```python
from build123d import *

# Parameters (mm, degrees)
F1_DEPTH = 203.2
F2_R     = 5.08
F4_DEPTH = 508
F5_R     = 17.4625
F6_DEPTH = 152.4
F8_DEPTH = 508


with BuildPart() as f1:
    # F0 (on Front) → F1 (new body)
    with BuildSketch(Plane.XZ):
        Polygon((-76.2, -46.21704), (-76.2, -57.094753), (76.2, -57.094753), (76.2, -46.21704), (26.83735, -33.72637), (21.163462, -31.835258), (18.708812, -29.612178), (16.218112, -26.55388), (14.689744, -22.895062), (13.485576, -19.143616), (13.305501, -16.85449), (10.935693, -2.660843), (9.173225, 23.941404), (9.095304, 51.274587), (9.465817, 61.371074), (10.203332, 68.52603), (11.415046, 73.405639), (12.987001, 77.66302), (14.984693, 80.446691), (18.095852, 83.001115), (20.683027, 84.147327), (25.922873, 85.98128), (30.180251, 87.1275), (33.094916, 87.749728), (34.175634, 88.306465), (35.387348, 89.616426), (36.173157, 90.991981), (36.40228, 91.97448), (36.598587, 93.513711), (36.598872, 93.52041), (36.827176, 98.88458), (36.669851, 103.667696), (36.407496, 106.64783), (36.177806, 110.315693), (35.555092, 114.278253), (34.24468, 117.978737), (33.327476, 119.878062), (31.132972, 122.464971), (28.218115, 124.036569), (24.026078, 125.34602), (19.539378, 126.000454), (15.433662, 126.392808), (7.999516, 126.762047), (0, 126.762047), (-7.999516, 126.762047), (-15.433662, 126.392808), (-19.539378, 126.000454), (-24.026078, 125.34602), (-28.218115, 124.036569), (-31.132972, 122.464971), (-33.327476, 119.878062), (-34.24468, 117.978737), (-35.555092, 114.278253), (-36.177806, 110.315693), (-36.407496, 106.64783), (-36.669851, 103.667696), (-36.827176, 98.88458), (-36.598872, 93.52041), (-36.598587, 93.513711), (-36.40228, 91.97448), (-36.173157, 90.991981), (-35.387348, 89.616426), (-34.175634, 88.306465), (-33.094916, 87.749728), (-30.180251, 87.1275), (-25.922873, 85.98128), (-20.683027, 84.147327), (-18.095852, 83.001115), (-14.984693, 80.446691), (-12.987001, 77.66302), (-11.415046, 73.405639), (-10.203332, 68.52603), (-9.465817, 61.371074), (-9.095304, 51.274587), (-9.173225, 23.941404), (-10.935693, -2.660843), (-13.305501, -16.85449), (-13.485576, -19.143616), (-14.689744, -22.895062), (-16.218112, -26.55388), (-18.708812, -29.612178), (-21.163462, -31.835258), (-26.83735, -33.72637), align=None)
    extrude(amount=F1_DEPTH)

    # F2
    f2_edges = [f1.edges().sort_by_distance(p)[0] for p in [
        (76.2, -101.6, -46.21704),
        (-76.2, -101.6, -46.21704),
    ]]
    fillet(f2_edges, radius=F2_R)

    # F3 (on face) → F4 (cut)
    with BuildSketch(Plane.XZ.offset(203.2)):
        with BuildLine():
            Line((26.83735, -33.72637), (21.163462, -31.835258))
            Line((21.163462, -31.835258), (21.163462, -57.094753))
            Line((21.163462, -57.094753), (76.2, -57.094753))
            Line((76.2, -57.094753), (76.2, -50.171713))
            ThreePointArc((76.2, -50.171713), (75.128547, -47.051144), (72.366162, -45.24693))
            Line((72.366162, -45.24693), (26.83735, -33.72637))
        make_face()
    extrude(amount=-F4_DEPTH, mode=Mode.SUBTRACT)

    # F5 (on Right) → F6 (cut, symmetric)
    with BuildSketch(Plane.YZ):
        with Locations((-101.6, 37.607995)):
            Circle(F5_R)
    extrude(amount=F6_DEPTH, both=True, mode=Mode.SUBTRACT)

    # F7 (on face) → F8 (cut)
    with BuildSketch(Plane.XZ.offset(203.2)):
        Polygon((15.433662, 126.392808), (7.999516, 126.762047), (36.669851, 103.667696), (36.407496, 106.64783), (36.177806, 110.315693), (35.555092, 114.278253), (34.24468, 117.978737), (33.327476, 119.878062), (31.132972, 122.464971), (28.218115, 124.036569), (24.026078, 125.34602), (19.539378, 126.000454), align=None)
    extrude(amount=-F8_DEPTH, mode=Mode.SUBTRACT)


solid = f1.part
```
The listing builds one solid part. Answer for the finished solid, in the listing's coordinates (mm). A direction names the side the tool comes from. Coordinates: 2 decimals unless noted, no trailing zeros. Write each loop counter-clockwise with the first axis right and the second up, starting at its lowest first coordinate (ties: lowest second). Pieces come first, ordered by that corner, then holes. Notation, with made-up numbers: M -16.75,3 L 2.25,3 A14 cw 2.25,17 Z; hole C -24,26 d6. An arc over 180 degrees is marked long. Use a Markdown table: item, result. Add a question column.
1. For a pull along Z with two mould halves and no side action, classify faces 5 (the flat face through (-8, -203.2, 36)), 6 (the flat face through (10.8, -100.18, 70.93)), 7 (the cylindrical face through (-75.16, -103.02, -47.09)) as +Z half, -Z half, draft (parallel to the pull), parting line (faces both ways), or undercut.
2. Straight lines are drawn through the part: line 1 along Z through (x, y) = (1.5, -101.6); line 2 along X through (y, z) = (-55.5, 41); line 3 along Z through (x, y) = (2, -101). For each, find the intervals that lie inside material, in ascending order. Write a range as [from, to].
3. Section A-A (x = -47.5) is taken. Give the vertices of the cut face in (y, z).
4. Section B-B (z = 1.5) is taken. Give the vertices of the cut face in (x, y), plus the area to 3 significant figures.
5. Which of the six approach directions +Z, -Z, +X, -X, +Y, -Y give full straight-line access (tool end or side, diameter ignored) to faces 1 (the flat face through (-21.75, -100.18, 125.68)), 2 (the flat face through (-49.283, -100.178, -39.406)), 3 (the flat face through (10.067, -100.178, 10.454)), 4 (the flat face through (21.163, -103, -44))?
6. Given P1, Ø2, axis at x = -24.5, y = -35, coming from the +Z side; P2, Ø2, axis at x = 17, z = -24, coming from the +Y side; P3, Ø5, axis at y = -55.5, z = 45.5, coming from the +X side; P4, Ø1, axis at y = -76.5, z = 105.5, coming from the -X side, each flat-ended and moving along its own axis, determine where each tip first touches the part or whether it passes through.
Data:
| question | item | result |
|---|---|---|
| 1 | face 5 | draft |
| 1 | face 6 | undercut |
| 1 | face 7 | +Z half |
| 2 | line 1 | z = [-57.09, 20.15], [55.07, 126.76] |
| 2 | line 2 | x = [-9.12, 9.12] |
| 2 | line 3 | z = [-57.09, 20.16], [55.06, 126.76] |
| 3 | outline | M -203.2,-57.09 L 0,-57.09 L 0,-38.95 L -203.2,-38.95 Z |
| 4 | outline | M -10.66,-203.2 L 10.66,-203.2 L 10.66,0 L -10.66,0 Z |
| 4 | area | 4,330 mm2 |
| 5 | face 1 | +Z, -X, +Y, -Y |
| 5 | face 2 | -X, +Y, -Y |
| 5 | face 3 | +X, +Y, -Y |
| 5 | face 4 | -Z, +X, +Y, -Y |
| 6 | P1 | stops at z = 125.42 |
| 6 | P2 | passes through |
| 6 | P3 | stops at x = 9.12 |
| 6 | P4 | stops at x = -36.55 |
